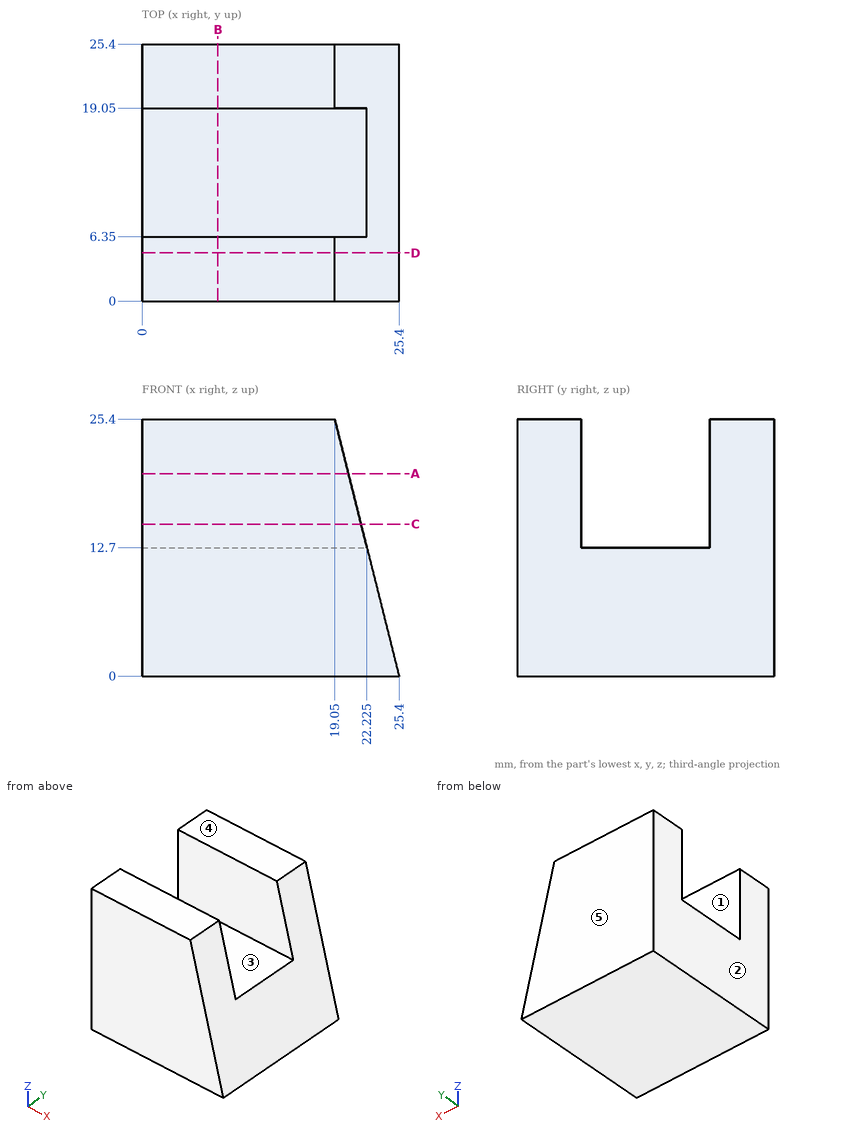
Design review of the part shown in the three views and the two pictorial views. Dimensions are in mm from the part's minimum x, y and z. A direction names the side the tool comes from. Round coordinates to 2 decimals unless told otherwise and drop trailing zeros. Loops run counter-clockwise (first coordinate to the right, second up) from the corner with the lowest first, then second, coordinate; pieces in that order, holes last. Notation, with made-up numbers: (-37, -17) - (1, -17) arc R17 ccw to (1, -1) - close; hole circle Ø4 at (41, 87.25). An arc over 180 degrees is marked (long way). Write each question's results on one line, items separated by ' | '. Start each with the question number.
Q1. Tool access review of the marked faces 1 and 2: name each direction out of +Z, -Z, +X, -X, +Y, -Y from which nothing blocks a thin tool from reaching the whole face with its end or side.
Q2. Take a section at B-B on x = 7.5. Give the boundary of the cut face in (y, z), plus the area to 3 significant figures.
Q3. Take a section at D-D on y = 4.75. Give the boundary of the cut face in (x, z).
Q4. Insertion check: P1, Ø2, axis at x = 15, y = 7.5, coming from the +Z side. The pin has a flat end and moves straight along its axis. Give the tip position at first contact, or say it passes through.
Q5. Take a section at A-A on z = 20. Give the boundary of the cut face in (x, y), plus the area to 3 significant figures.
Q6. Draft analysis for pull direction Y (two halves, no side actions). For the marked faces 3, 4 and 5, state which applies: pulls with the +Y half, pulls with the -Y half, needs draft (parallel to the pull), parting line crosses it, or undercut.
Q7. Take a section at C-C on z = 15. Give the boundary of the cut face in (x, y), plus the area to 3 significant figures.
Q8. Wall thickness on line 1 along Y through (x, z) = (9.5, 23.5); line 2 along Z through (x, y) = (19, 9.75); line 3 along X through (y, z) = (10.25, 3.25): over which ranges is each line inside the solid? List them lowest first. Write a range as [from, to].
Data:
1) face 1: +Z, +X, -X | face 2: +Z, -Z, -X, +Y, -Y
2) outline: (0, 0) - (25.4, 0) - (25.4, 25.4) - (19.05, 25.4) - (19.05, 12.7) - (6.35, 12.7) - (6.35, 25.4) - (0, 25.4) - close | area: 484 mm²
3) outline: (0, 0) - (25.4, 0) - (19.05, 25.4) - (0, 25.4) - close
4) P1: stops at z = 12.7
5) outline: (0, 0) - (20.4, 0) - (20.4, 6.35) - (0, 6.35) - close; (0, 19.05) - (20.4, 19.05) - (20.4, 25.4) - (0, 25.4) - close | area: 259 mm²
6) face 3: undercut | face 4: needs draft | face 5: pulls with the +Y half
7) outline: (0, 0) - (21.65, 0) - (21.65, 6.35) - (0, 6.35) - close; (0, 19.05) - (21.65, 19.05) - (21.65, 25.4) - (0, 25.4) - close | area: 275 mm²
8) line 1: y = [0, 6.35], [19.05, 25.4] | line 2: z = [0, 12.7] | line 3: x = [0, 24.59]
